from build123d import *

# Parameters (mm, degrees)
SKETCH1_W               = 23.6
SKETCH1_H               = 8.6
BOSS_EXTRUDE1_DEPTH     = 22
SKETCH2_W               = 14.6
SKETCH2_H               = 29.6
BOSS_EXTRUDE2_DEPTH     = 130
SKETCH3_R               = 1.7
CUT_EXTRUDE1_DEPTH      = 9
CUT_EXTRUDE2_DEPTH      = 154.533959474
CUT_EXTRUDE2_DEPTH_BACK = 19
SKETCH5_R               = 2.06
BOSS_EXTRUDE3_DEPTH     = 9


with BuildPart() as part:
    # Sketch1 → Boss-Extrude1 (new body)
    with BuildSketch(Plane(origin=(0, 0, 0), x_dir=(0, 1, 0), z_dir=(0, 0, 1))):
        with Locations((-1.18489011, 2.334615385)):
            Rectangle(SKETCH1_W, SKETCH1_H)
    extrude(amount=BOSS_EXTRUDE1_DEPTH)

    # Sketch2 → Boss-Extrude2 (add)
    with BuildSketch(Plane.XY.offset(22)):
        with Locations((-2.334615385, -1.18489011)):
            Rectangle(SKETCH2_W, SKETCH2_H)
    extrude(amount=BOSS_EXTRUDE2_DEPTH)

    # Sketch3 → Cut-Extrude1 (cut)
    with BuildSketch(Plane.YZ.offset(1.965384615)):
        with Locations(Location((6.81510989, 5.3, 0), (0, 0, 270))):
            Circle(SKETCH3_R)
        with Locations(Location((-9.18489011, 5.3, 0), (0, 0, 270))):
            Circle(SKETCH3_R)
    extrude(amount=-CUT_EXTRUDE1_DEPTH, mode=Mode.SUBTRACT)

    # Sketch4 → Cut-Extrude2 (cut, two sides: drawn at the far end of the back side and taken through both)
    with BuildSketch(Plane.YZ.offset(4.965384615).offset(-CUT_EXTRUDE2_DEPTH_BACK)):
        Polygon((-4.013317235, 118.028427125), (-10.98489011, 125), (-10.98489011, 111.056854249), align=None)
        Polygon((4.958255641, 127), (-7.32803586, 127), (-1.18489011, 120.856854249), align=None)
        Polygon((8.61510989, 125), (1.643537015, 118.028427125), (8.61510989, 111.056854249), align=None)
        Polygon((-1.18489011, 115.2), (-8.156462985, 108.228427125), (-1.18489011, 101.256854249), (5.786682765, 108.228427125), align=None)
        Polygon((-4.013317235, 98.428427125), (-10.98489011, 105.4), (-10.98489011, 91.456854249), align=None)
        Polygon((8.61510989, 105.4), (1.643537015, 98.428427125), (8.61510989, 91.456854249), align=None)
        Polygon((-1.18489011, 95.6), (-8.156462985, 88.628427125), (-1.18489011, 81.656854249), (5.786682765, 88.628427125), align=None)
        Polygon((-4.013317235, 78.828427125), (-10.98489011, 85.8), (-10.98489011, 71.856854249), align=None)
        Polygon((8.61510989, 85.8), (1.643537015, 78.828427125), (8.61510989, 71.856854249), align=None)
        Polygon((-1.18489011, 76), (-8.156462985, 69.028427125), (-1.18489011, 62.056854249), (5.786682765, 69.028427125), align=None)
        Polygon((-10.98489011, 66.2), (-10.98489011, 52.256854249), (-4.013317235, 59.228427125), align=None)
        Polygon((1.643537015, 59.228427125), (8.61510989, 52.256854249), (8.61510989, 66.2), align=None)
        Polygon((-1.18489011, 56.4), (-8.156462985, 49.428427125), (-1.18489011, 42.456854249), (5.786682765, 49.428427125), align=None)
        Polygon((-10.98489011, 46.6), (-10.98489011, 32.656854249), (-4.013317235, 39.628427125), align=None)
        Polygon((1.643537015, 39.628427125), (8.61510989, 32.656854249), (8.61510989, 46.6), align=None)
        Polygon((-1.18489011, 36.8), (-10.98489011, 27), (8.61510989, 27), align=None)
        Polygon((-8.156462985, 127.828427125), (-7.32803586, 127), (4.958255641, 127), (5.786682765, 127.828427125), (-1.18489011, 134.8), align=None)
        Polygon((-10.98489011, 144.6), (-10.98489011, 130.656854249), (-4.013317235, 137.628427125), align=None)
        Polygon((-8.98489011, 148.256854249), (-1.18489011, 140.456854249), (6.61510989, 148.256854249), align=None)
        Polygon((8.61510989, 144.6), (1.643537015, 137.628427125), (8.61510989, 130.656854249), align=None)
    extrude(amount=CUT_EXTRUDE2_DEPTH + CUT_EXTRUDE2_DEPTH_BACK, mode=Mode.SUBTRACT)

    # Sketch5 → Boss-Extrude3 (add)
    # profile 1 of 3: a face of its own
    with BuildSketch(Plane.YZ.offset(4.965384615)):
        with BuildLine():
            Line((-15.98489011, 155.72240804), (-15.98489011, 152))
            Line((-15.98489011, 152), (-10.3500415, 152))
            ThreePointArc((-10.3500415, 152), (-13.311150898, 153.643698648), (-15.98489011, 155.72240804))
        make_face()
    # profile 2 of 3: a face of its own
    with BuildSketch(Plane.YZ.offset(4.965384615)):
        with BuildLine():
            ThreePointArc((13.61510989, 155.72240804), (10.941370678, 153.643698648), (7.98026128, 152))
            Line((7.98026128, 152), (13.61510989, 152))
            Line((13.61510989, 152), (13.61510989, 155.72240804))
        make_face()
    # profile 3 of 3: a face of its own
    with BuildSketch(Plane.YZ.offset(4.965384615)):
        with BuildLine():
            ThreePointArc((20.81510989, 172), (-10.084328294, 192.119642144), (-15.98489011, 155.72240804))
            ThreePointArc((-15.98489011, 155.72240804), (-13.311150898, 153.643698648), (-10.3500415, 152))
            Line((-10.3500415, 152), (7.98026128, 152))
            ThreePointArc((7.98026128, 152), (10.941370678, 153.643698648), (13.61510989, 155.72240804))
            ThreePointArc((13.61510989, 155.72240804), (18.934752034, 163.100561815), (20.81510989, 172))
        make_face()
        with Locations((-13.20570539, 159.97918472)):
            Circle(SKETCH5_R, mode=Mode.SUBTRACT)
        with Locations((-13.20570539, 184.02081528)):
            Circle(SKETCH5_R, mode=Mode.SUBTRACT)
        with Locations((10.83592517, 159.97918472)):
            Circle(SKETCH5_R, mode=Mode.SUBTRACT)
        with Locations((10.83592517, 184.02081528)):
            Circle(SKETCH5_R, mode=Mode.SUBTRACT)
    extrude(amount=-BOSS_EXTRUDE3_DEPTH)


solid = part.part
Build history of the part. All positions in model axes, mm. A direction names the side the tool comes from. Coordinates: 2 decimals unless noted, no trailing zeros. Write each loop counter-clockwise with the first axis right and the second up, starting at its lowest first coordinate (ties: lowest second). Pieces come first, ordered by that corner, then holes. Notation, with made-up numbers: (53, 33.25) -> (58, 33.25) arc R9 cw to (58, 47.25) -> close; hole circle Ø4 at (42, 69). An arc over 180 degrees is marked (long way). Use CSV: the item, a comma, the result in double quotes. Start each with the question number.
Q1. Flat gauge pins, fed straight in: pin 1 Ø4 at (x, z) = (-2.5, 137.5) entering from -Y; pin 2 Ø6 at (x, y) = (-5.5, -4.5) entering from +Z; pin 3 Ø7 at (x, z) = (-2.5, 78.5) entering from +Y; pin 4 Ø3.5 at (y, z) = (-13.21, 184.02) entering from -X. Where does each tip first touch, or does it go through?
Q2. Pull direction Z, two halves, no side cores. Call faces 1 (the flat face through (-4.035, -1, 173)), 2 (the flat face through (-2, 8.615, 59)): released by +Z, released by -Z, zero draft, split by the parting line, or undercut.
Q3. Cut at D-D, the plane z = 165.5. List the corners of the cut face in (x, y).
Q4. Cut at A-A, the plane z = 5.3. List the corners of the cut face in (x, y).
Q5. Cut at C-C, the plane y = 18. List the corners of the cut face in (x, z).
Q6. 3-axis set-ups, long thin cutter, end or side, ignore diameter. For faces 3 (the flat face through (-2, -10.985, 40)), 4 (the flat face through (-2, 13.615, 88)), 5 (the flat face through (4.965, 8, 109)): which of +Z, -Z, +X, -X, +Y, -Y reach the whole face in a straight line?
Q7. Cut at B-B, the plane z = 132.5. List the corners of the cut face in (x, y).
Q8. Drill centre lines: probe 1 along Y at (x, z) = (-2.75, 5.3); probe 2 along Y at (x, z) = (1.5, 118); probe 3 along Z at (x, y) = (3.25, 9.5). Where is each one in solid material? Low to high.
Checked values:
1,pin 1,"stops at y = -15.98"
1,pin 2,"stops at z = 193.99"
1,pin 3,"stops at y = 13.62"
1,pin 4,"passes through"
2,face 1,"zero draft"
2,face 2,"undercut"
3,outline,"(-4.03, -22.2) -> (4.97, -22.2) -> (4.97, 19.83) -> (-4.03, 19.83) -> close"
4,outline,"(-6.63, -12.98) -> (1.97, -12.98) -> (1.97, -10.88) -> (-6.63, -10.88) -> close; (-6.63, -7.48) -> (1.97, -7.48) -> (1.97, 5.12) -> (-6.63, 5.12) -> close; (-6.63, 8.52) -> (1.97, 8.52) -> (1.97, 10.62) -> (-6.63, 10.62) -> close"
5,outline,"(-4.03, 161.23) -> (4.97, 161.23) -> (4.97, 182.77) -> (-4.03, 182.77) -> close"
6,face 3,"+X, -X"
6,face 4,"-Z, +X, -X, +Y"
6,face 5,"+Z, -Z, +X, +Y, -Y"
7,outline,"(-9.63, -15.98) -> (4.97, -15.98) -> (4.97, -10.98) -> (-9.63, -10.98) -> close; (-9.63, -9.14) -> (4.97, -9.14) -> (4.97, -3.48) -> (-9.63, -3.48) -> close; (-9.63, 1.12) -> (4.97, 1.12) -> (4.97, 6.77) -> (-9.63, 6.77) -> close; (-9.63, 8.62) -> (4.97, 8.62) -> (4.97, 13.62) -> (-9.63, 13.62) -> close"
8,probe 1,"y = -12.98 to -10.88, -7.48 to 5.12, 8.52 to 10.62"
8,probe 2,"y = -15.98 to -10.98, -4.04 to 1.67, 8.62 to 13.62"
8,probe 3,"z = 22 to 158.41, 161.55 to 182.45, 185.59 to 191.23"
